Autodesk Inventor part; units mm, degrees
ref_plane "YZ Plane" through (0, 0, 0) normal (1, 0, 0) x (0, 1, 0)
ref_plane "XZ Plane" through (0, 0, 0) normal (0, 1, 0) x (-1, 0, 0)
ref_plane "XY Plane" through (0, 0, 0) normal (0, 0, 1) x (1, 0, 0)
sketch "Esquisse1" plane through (0, 0, 0) normal (0, 1, 0) x (-1, 0, 0)
  circle A0 centre (0, 0) radius 2.5
  dimension "d0" = 5
extrude "Extrusion1" add sketch "Esquisse1" along normal mid plane 5
sketch "Esquisse2" plane through (0, -2.5, 0) normal (0, -1, 0) x (1, 0, 0)
  circle A0 centre (0, 0) radius 2
  dimension "d3" = 4
extrude "Extrusion2" add sketch "Esquisse2" along normal blind 4
thread "Filetage1"
chamfer "Chanfrein1" distance 0.5 angle 45 1 edges at (-2, -6.5, 0)
mirror "Symétrie1" about plane through (0, 0, 0) normal (0, 1, 0) of "Extrusion2", "Chanfrein1"
properties part number "tige_serrage_main" material "Aluminium 6061"
The listing builds one solid part. Answer for the finished solid, in the listing's coordinates (mm). A direction names the side the tool comes from. Give positions to 0.01 mm unless a question says otherwise; leave off trailing zeros. Loops run counter-clockwise (first coordinate to the right, second up) from the corner with the lowest first, then second, coordinate; pieces in that order, holes last. Notation, with made-up numbers: (56, -15.5) - (110, -15.5) arc R15 cw to (110, 0.5) - close; hole circle Ø2 at (24.25, 51). An arc over 180 degrees is marked (long way). Answer as a JSON object with one key per item and string values.
1. Find the intervals of material crossed by L1, parallel to X at y = -2, z = 1.5; L2, parallel to Z at x = 0.2, y = -4.5; L3, parallel to Y at x = 0.9, z = 1.85, in increasing order. Write a range as [from, to].
Determined:
{"L1": "[-2, 2]", "L2": "[-1.99, 1.99]", "L3": "[-2.5, 2.5]"}
2. A cutting plane is placed at D-D (z = 2.2). Write down the section's boundary in (x, y), then the cut area to 3 significant figures.
Determined:
{"outline": "(-1.19, -2.5) - (1.19, -2.5) - (1.19, 2.5) - (-1.19, 2.5) - close", "area": "11.9 mm²"}
3. A cutting plane is placed at C-C (y = 0.25). Write down the section's boundary in (x, z).
Determined:
{"outline": "circle Ø5 at (0, 0)"}
4. For a pull along X with two mould halves and no side action, classify faces 3 (the flat face through (1, 2.5, 2)), 4 (the cylindrical face through (0, 4, -2)) as pulls with the +X half, pulls with the -X half, needs draft (parallel to the pull), parting line crosses it, or undercut.
Determined:
{"face 3": "needs draft", "face 4": "parting line crosses it"}
5. A cutting plane is placed at A-A (z = 0). Write down the section's boundary in (x, y), then the cut area to 3 significant figures.
Determined:
{"outline": "(-2.5, -2.5) - (-2, -2.5) - (-2, -6) - (-1.5, -6.5) - (1.5, -6.5) - (2, -6) - (2, -2.5) - (2.5, -2.5) - (2.5, 2.5) - (2, 2.5) - (2, 6) - (1.5, 6.5) - (-1.5, 6.5) - (-2, 6) - (-2, 2.5) - (-2.5, 2.5) - close", "area": "56.5 mm²"}
6. For faces 1 (the flat face through (0, 6.5, 0)), 2 (the flat face through (1, -2.5, 2)), determine the directions among +Z, -Z, +X, -X, +Y, -Y from which every point of the face is accessible in a straight line to the end or side of a thin tool.
Determined:
{"face 1": "+Z, -Z, +X, -X, +Y", "face 2": "-Y"}
7. A cutting plane is placed at B-B (x = 0). Write down the section's boundary in (y, z), then the cut area to 3 significant figures.
Determined:
{"outline": "(-6.5, -1.5) - (-6, -2) - (-2.5, -2) - (-2.5, -2.5) - (2.5, -2.5) - (2.5, -2) - (6, -2) - (6.5, -1.5) - (6.5, 1.5) - (6, 2) - (2.5, 2) - (2.5, 2.5) - (-2.5, 2.5) - (-2.5, 2) - (-6, 2) - (-6.5, 1.5) - close", "area": "56.5 mm²"}
